Read the model definition and answer for the solid it produces. Units are mm, in the model's axes. A direction names the side the tool comes from. Coordinates: 2 decimals unless noted, no trailing zeros. Write each loop counter-clockwise with the first axis right and the second up, starting at its lowest first coordinate (ties: lowest second). Pieces come first, ordered by that corner, then holes. Notation, with made-up numbers: (37.25, 68) -> (70.25, 68) arc R27 ccw to (70.25, 90) -> close; hole circle Ø4 at (-22.75, -22.75). An arc over 180 degrees is marked (long way). Answer in a Markdown table with one row per item. Add a question column.
Item 1: For a pull along Y with two mould halves and no side action, classify faces 1 (the face through (-2, -2, 0)), 2 (the face through (1.987, -0.626, 18.533)), 3 (the face through (-1.03, 0.6, -1.43)) as +Y half, -Y half, draft (parallel to the pull), parting line (faces both ways), or undercut.
Item 2: Which of the six approach directions +Z, -Z, +X, -X, +Y, -Y give full straight-line access (tool end or side, diameter ignored) to faces 4 (the face through (1.036, 0.587, -1.427)), 5 (the face through (0, 0, 38.1))?
Item 3: Given pin 1 Ø0.7 at (x, z) = (0, -1.5) entering from -Y; pin 2 Ø1 at (y, z) = (-0.5, 33.5) entering from -X; pin 3 Ø4 at (y, z) = (1, 5.5) entering from +X; pin 4 Ø2.5 at (x, y) = (-1, 2) entering from +Z, each flat-ended and moving along its own axis, determine where each tip first touches the part or whether it passes through.
Item 4: Straight lines are drawn through the part: line 1 (Y direction, x = 0, z = 15); line 2 (Z direction, x = 2.75, y = -1.25); line 3 (X direction, y = 0.25, z = -1). For each, find the intervals that lie inside material, in ascending order. Write a range as from..to.
Item 5: Section A-A on z = 14.5 is taken. Write down the section's boundary in (x, y).
Autodesk Inventor part; units mm, degrees
ref_plane "YZ Plane" through (0, 0, 0) normal (1, 0, 0) x (0, 1, 0)
ref_plane "XZ Plane" through (0, 0, 0) normal (0, 1, 0) x (-1, 0, 0)
ref_plane "XY Plane" through (0, 0, 0) normal (0, 0, 1) x (1, 0, 0)
sketch "Sketch1" plane through (0, 0, 0) normal (0, 0, 1) x (1, 0, 0)
  circle A0 centre (0, 0) radius 2.0828
  dimension "d0" = 4.1656
extrude "Extrusion1" add sketch "Sketch1" along normal blind 38.1
sketch "Sketch2" plane through (0, 0, 0) normal (0, 1, 0) x (-1, 0, 0)
  line L0 (0, 0) -> (0, -2.2098)
  line L1 (0, 0) -> (3.9624, 0)
  line L2 (0, -2.2098) -> (2.032, -2.2098)
  line L3 (3.9624, 0) -> (3.9624, 3.6562) construction
  arc A0 (2.032, -2.2098) -> (3.9624, -0.4599) centre (0.1837, 1.7689) ccw
  line L4 (4.5847, 0.6553) -> (4.5847, -0.2608) construction
  line L5 (3.9624, -0.4599) -> (3.9624, 0)
  dimension "d3" = 2.2098
  dimension "d6" = 2.032
  dimension "d19" = 3.9624
revolve "Revolution1" add sketch "Sketch2" angle 360 about axis through (0, 0, 0) along (0, 0, -1)
sketch "Sketch3" plane through (0, 0, -2.2098) normal (0, 0, -1) x (-1, 0, 0)
  circle A0 centre (0, 0) radius 2.032
  line L0 (-0.6874, 1.1906) -> (0.6874, 1.1906)
  line L1 (0.6874, 1.1906) -> (1.3748, 0)
  line L2 (1.3748, 0) -> (0.6874, -1.1906)
  line L3 (0.6874, -1.1906) -> (-0.6874, -1.1906)
  line L4 (-0.6874, -1.1906) -> (-1.3748, 0)
  line L5 (-1.3748, 0) -> (-0.6874, 1.1906)
  dimension "d8" = 2.3813
extrude "Extrusion2" cut sketch "Sketch3" against normal blind 1.5875 contours L0 L1 L2 L3 L4 L5
chamfer "Chamfer1" distance 0.508 angle 45 1 edges at (-2.0828, 0, 38.1)
thread "Thread1"
properties part number "10-32 x500 button head" material "Aluminum 6061"
Results below:
| question | item | result |
|---|---|---|
| 1 | face 1 | draft |
| 1 | face 2 | parting line |
| 1 | face 3 | undercut |
| 2 | face 4 | -Z |
| 2 | face 5 | +Z, +X, -X, +Y, -Y |
| 3 | pin 1 | stops at y = -3.46 |
| 3 | pin 2 | stops at x = -2.08 |
| 3 | pin 3 | stops at x = 2.08 |
| 3 | pin 4 | stops at z = 38.1 |
| 4 | line 1 | y = -2.08..2.08 |
| 4 | line 2 | z = -1.58..0 |
| 4 | line 3 | x = -3.58..-1.23, 1.23..3.58 |
| 5 | outline | circle Ø4.17 at (0, 0) |
